For this review, take the finished solid that the model builds, in its own axes (mm). A direction names the side the tool comes from. Give positions to 0.01 mm unless a question says otherwise; leave off trailing zeros. Write each loop counter-clockwise with the first axis right and the second up, starting at its lowest first coordinate (ties: lowest second). Pieces come first, ordered by that corner, then holes. Notation, with made-up numbers: M 17.5,60 L 54.5,60 A20 cw 54.5,68 Z; hole C 25,45 d10. An arc over 180 degrees is marked long. Write item = value, one per line.
```python
from build123d import *

# Parameters (mm, degrees)
SKETCH1_R           = 31.5
BOSS_EXTRUDE1_DEPTH = 42
SKETCH2_R           = 31.5
BOSS_EXTRUDE2_DEPTH = 6
CHAMFER1_SIZE       = 6
SKETCH4_R           = 31.5
BOSS_EXTRUDE3_DEPTH = 8
CHAMFER2_SIZE       = 8
SKETCH6_R           = 7.5
BOSS_EXTRUDE4_DEPTH = 1
SKETCH7_R           = 4
BOSS_EXTRUDE5_DEPTH = 24
SKETCH10_R          = 2
CUT_EXTRUDE4_DEPTH  = 8
CUT_EXTRUDE5_DEPTH  = 10
SKETCH12_R          = 10.5
SKETCH12_R_2        = 6.5
CUT_EXTRUDE6_DEPTH  = 2


with BuildPart() as part:
    # Sketch1 → Boss-Extrude1 (new body)
    with BuildSketch(Plane.XY):
        with Locations(Location((0, 0, 0), (0, 0, 180))):
            Circle(SKETCH1_R)
    extrude(amount=BOSS_EXTRUDE1_DEPTH)

    # Sketch2 → Boss-Extrude2 (add)
    with BuildSketch(Plane.XY.offset(42)):
        with Locations(Location((0, 0, 0), (0, 0, 180))):
            Circle(SKETCH2_R)
    extrude(amount=BOSS_EXTRUDE2_DEPTH)

    # Chamfer1
    chamfer1_edges = [part.edges().sort_by_distance(p)[0] for p in [
        (31.5, 0, 48),
    ]]
    chamfer(chamfer1_edges, length=CHAMFER1_SIZE)

    # Sketch4 → Boss-Extrude3 (add)
    with BuildSketch(Plane(origin=(0, 0, 0), x_dir=(-1, 0, 0), z_dir=(0, 0, -1))):
        Circle(SKETCH4_R)
    extrude(amount=BOSS_EXTRUDE3_DEPTH)

    # Chamfer2
    chamfer2_edges = [part.edges().sort_by_distance(p)[0] for p in [
        (31.5, 0, -8),
    ]]
    chamfer(chamfer2_edges, length=CHAMFER2_SIZE)

    # Sketch6 → Boss-Extrude4 (add)
    with BuildSketch(Plane(origin=(0, 0, -8), x_dir=(-1, 0, 0), z_dir=(0, 0, -1))):
        Circle(SKETCH6_R)
    extrude(amount=BOSS_EXTRUDE4_DEPTH)

    # Sketch7 → Boss-Extrude5 (add)
    with BuildSketch(Plane.XY.offset(48)):
        Circle(SKETCH7_R)
    extrude(amount=BOSS_EXTRUDE5_DEPTH)

    # Sketch10 → Cut-Extrude4 (cut)
    with BuildSketch(Plane.XY.offset(48)):
        with Locations((0, 15.2)):
            Circle(SKETCH10_R)
        with Locations((0, 22.2)):
            Circle(SKETCH10_R)
        with Locations((22.2, 0)):
            Circle(SKETCH10_R)
        with Locations((15.2, 0)):
            Circle(SKETCH10_R)
        with Locations((0, -22.2)):
            Circle(SKETCH10_R)
        with Locations((0, -15.2)):
            Circle(SKETCH10_R)
        with Locations((-22.2, 0)):
            Circle(SKETCH10_R)
        with Locations((-15.2, 0)):
            Circle(SKETCH10_R)
    extrude(amount=-CUT_EXTRUDE4_DEPTH, mode=Mode.SUBTRACT)

    # Sketch11 → Cut-Extrude5 (cut)
    with BuildSketch(Plane(origin=(2.5, 0, 0), x_dir=(0, 0, -1), z_dir=(1, 0, 0))):
        with BuildLine():
            Line((-67.418537693, 1.5), (-53.527084748, 1.5))
            ThreePointArc((-53.527084748, 1.5), (-52.027084748, 0), (-53.527084748, -1.5))
            Line((-53.527084748, -1.5), (-67.418537693, -1.5))
            ThreePointArc((-67.418537693, -1.5), (-68.918537693, 0), (-67.418537693, 1.5))
        make_face()
    extrude(amount=CUT_EXTRUDE5_DEPTH, mode=Mode.SUBTRACT)

    # Sketch12 → Cut-Extrude6 (cut)
    with BuildSketch(Plane.XY.offset(48)):
        Circle(SKETCH12_R)
        Circle(SKETCH12_R_2, mode=Mode.SUBTRACT)
    extrude(amount=-CUT_EXTRUDE6_DEPTH, mode=Mode.SUBTRACT)


solid = part.part
```
1. Machinability: for faces 4 (the face through (7.493, 0.33, -8.493)), 5 (the face through (0, 0, -9)), 6 (the face through (-15, 0, 40)), which of the approach directions +Z, -Z, +X, -X, +Y, -Y give a long, thin tool a straight path to every point of the face, cutting with its end or side? Answer none if there is none.
Responses:
face_4 = -Z
face_5 = -Z, +X, -X, +Y, -Y
face_6 = +Z
2. Insertion check: P1, Ø6, axis at x = 20.5, z = 17.5, coming from the -Y side; P2, Ø2.5, axis at x = -15.2, y = 0, coming from the +Z side; P3, Ø3, axis at x = 0.5, y = 15.5, coming from the +Z side. Each pin has a flat end and moves straight along its axis. Give the tip position at first contact, or say it passes through.
Responses:
P1 = -26.19
P2 = 40
P3 = 48
3. For line 1 along Y through (x, z) = (0, 44); line 2 along Y through (x, z) = (0, 43); line 3 along Z through (x, y) = (8.5, 18.5), list the stretches that pass through material, from the lowest coordinate up. Write a range as from..to.
Responses:
line_1 = -29.5..-24.2, -20.2..-17.2, -13.2..13.2, 17.2..20.2, 24.2..29.5
line_2 = -30.5..-24.2, -20.2..-17.2, -13.2..13.2, 17.2..20.2, 24.2..30.5
line_3 = -8..48
4. The part is to be moulded in two halves that separate along Y. For faces 1 (the face through (-3, -3, 48)), 2 (the face through (5.591, 25.178, 47.709)), 3 (the face through (-22, 0, 40)), say which applies: +Y half, -Y half, draft (parallel to the pull), parting line (faces both ways), or undercut.
Responses:
face_1 = draft
face_2 = parting line
face_3 = undercut
5. We need section B-B, the plane z = 60. Write out the cut boundary in (x, y), then the cut area to 3 significant figures.
Responses:
outline = M 2.5,-1.5 L 2.5,1.5 L 3.71,1.5 A4 ccw long 3.71,-1.5 Z
area = 46.1 mm2
6. We need section A-A, the plane z = 11. Write out the cut boundary in (x, y).
Responses:
outline = C 0,0 d63
